from build123d import *

# Parameters (mm, degrees)
SKETCH_1_R          = 24
SKETCH_1_R_2        = 2
SKETCH_1_R_3        = 2.5
SKETCH_1_R_4        = 1.1
SKETCH_1_R_5        = 6
EXTRUDE_1_DEPTH     = 6
SKETCH_2_R          = 1
CUT_EXTRUDE_1_DEPTH = 84.432607534
FILLET_1_R          = 1


with BuildPart() as part:
    # 草图1 → 凸台-拉伸1 (new body)
    with BuildSketch(Plane.XY):
        with BuildLine():
            Line((-31, 0), (-31, 44.038518603))
            ThreePointArc((-31, 44.038518603), (-32.603168898, 47.707515532), (-36.384615385, 49.023703756))
            ThreePointArc((-36.384615385, 49.023703756), (-44.994071865, 56.692079518), (-37, 65))
            Line((-37, 65), (-12.5, 65))
            Line((-12.5, 65), (-12.5, 70))
            Line((-12.5, 70), (12.5, 70))
            Line((12.5, 70), (12.5, 65))
            Line((12.5, 65), (31, 65))
            Line((31, 65), (31, 0))
            ThreePointArc((31, 0), (24.191352338, -19.385006373), (6.756227609, -30.254807692))
            ThreePointArc((6.756227609, -30.254807692), (5.147421514, -30.170867126), (3.813999457, -29.266826923))
            ThreePointArc((3.813999457, -29.266826923), (0, -27.5), (-3.813999457, -29.266826923))
            ThreePointArc((-3.813999457, -29.266826923), (-5.147421514, -30.170867126), (-6.756227609, -30.254807692))
            ThreePointArc((-6.756227609, -30.254807692), (-24.191352338, -19.385006373), (-31, 0))
        make_face()
        Circle(SKETCH_1_R, mode=Mode.SUBTRACT)
        with Locations((-19.445436483, 19.445436483)):
            Circle(SKETCH_1_R_2, mode=Mode.SUBTRACT)
        with Locations((0, 27.5)):
            Circle(SKETCH_1_R_2, mode=Mode.SUBTRACT)
        with Locations((19.445436483, 19.445436483)):
            Circle(SKETCH_1_R_2, mode=Mode.SUBTRACT)
        with Locations((27.5, 0)):
            Circle(SKETCH_1_R_2, mode=Mode.SUBTRACT)
        with Locations((19.445436483, -19.445436483)):
            Circle(SKETCH_1_R_2, mode=Mode.SUBTRACT)
        with Locations((-19.445436483, -19.445436483)):
            Circle(SKETCH_1_R_2, mode=Mode.SUBTRACT)
        with Locations((-27.5, 0)):
            Circle(SKETCH_1_R_2, mode=Mode.SUBTRACT)
        with Locations((-26, 60)):
            Circle(SKETCH_1_R_3, mode=Mode.SUBTRACT)
        with Locations((0, 60)):
            Circle(SKETCH_1_R_3, mode=Mode.SUBTRACT)
        with Locations((26, 60)):
            Circle(SKETCH_1_R_3, mode=Mode.SUBTRACT)
        with Locations((-22.6, 50)):
            Circle(SKETCH_1_R_4, mode=Mode.SUBTRACT)
        with Locations((-22.6, 32)):
            Circle(SKETCH_1_R_4, mode=Mode.SUBTRACT)
        with Locations((22.6, 32)):
            Circle(SKETCH_1_R_4, mode=Mode.SUBTRACT)
        with Locations((22.6, 50)):
            Circle(SKETCH_1_R_4, mode=Mode.SUBTRACT)
        with Locations((-37, 57)):
            Circle(SKETCH_1_R_5, mode=Mode.SUBTRACT)
    extrude(amount=EXTRUDE_1_DEPTH)

    # 草图2 → 切除-拉伸1 (cut, through all)
    with BuildSketch(Plane.XY.offset(6)):
        with Locations((-13.5, 65)):
            Circle(SKETCH_2_R)
        with Locations((13.5, 65)):
            Circle(SKETCH_2_R)
    extrude(amount=-CUT_EXTRUDE_1_DEPTH, mode=Mode.SUBTRACT)

    # 圆角1
    fillet_1_edges = [part.edges().sort_by_distance(p)[0] for p in [
        (-12.5, 70, 3),
        (12.5, 70, 3),
        (31, 65, 3),
    ]]
    fillet(fillet_1_edges, radius=FILLET_1_R)


solid = part.part
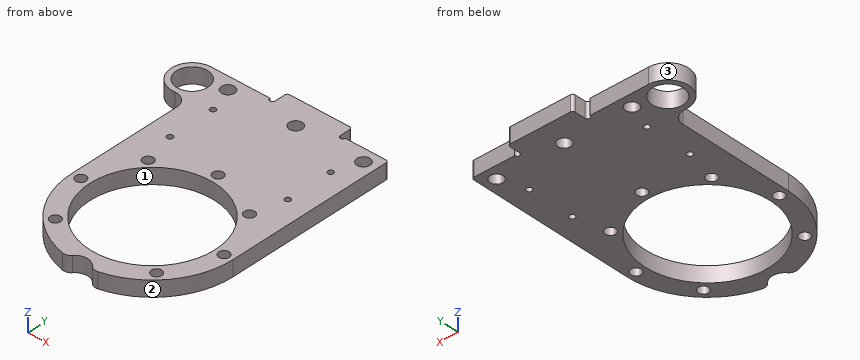
Input: part model. Units: mm. Frame: model coordinates. Face numbers are marked on the shaded views. Round coordinates to 2 decimals unless told otherwise and drop trailing zeros. Write each loop counter-clockwise with the first axis right and the second up, starting at its lowest first coordinate (ties: lowest second). Pieces come first, ordered by that corner, then holes.
1) Contact query for flat-ended pins moving along their axis: P1, Ø3, axis at x = -27.5, y = 0, coming from the -Z side; P2, Ø1.8, axis at x = -30, z = 2, coming from the +Y side; P3, Ø1, axis at x = -32, z = 1.5, coming from the -Y side; P4, Ø1, axis at y = 58.5, z = 2.5, coming from the -X side. Output: stop coordinate, or through.
2) Draft query along Y for the marked faces 1, 2 and 3. Return one class per face: pulls with the +Y half, pulls with the -Y half, needs draft (parallel to the pull), parting line crosses it, or undercut.
3) Cut plane C-C (x = -8.5). Return the cut outline in (y, z), then the cut area to 3 significant figures.
4) Cut plane D-D (y = 60). Return the cut outline in (x, z).
5) Cut plane B-B (x = 0). Return the cut outline in (y, z), then the cut area to 3 significant figures.
6) Cut plane A-A (y = 32). Return the cut outline in (x, z).
7) Ray query, L1, parallel to X at y = 21, z = 1.7; L2, parallel to Y at x = -18.5, z = 5.5; L3, parallel to X at y = 1, z = 5.6. Return the intervals inside material, ascending.
Geometry says:
1. P1: passes through
1. P2: stops at y = 65
1. P3: stops at y = 46.22
1. P4: stops at x = -44.94
2. face 1: undercut
2. face 2: pulls with the -Y half
2. face 3: parting line crosses it
3. outline: (-29.81, 0) - (-22.44, 0) - (-22.44, 6) - (-29.81, 6) - close; (22.44, 0) - (70, 0) - (70, 6) - (22.44, 6) - close
3. area: 330 mm2
4. outline: (-44.42, 0) - (-42.2, 0) - (-42.2, 6) - (-44.42, 6) - close; (-31.8, 0) - (-28.5, 0) - (-28.5, 6) - (-31.8, 6) - close; (-23.5, 0) - (-2.5, 0) - (-2.5, 6) - (-23.5, 6) - close; (2.5, 0) - (23.5, 0) - (23.5, 6) - (2.5, 6) - close; (28.5, 0) - (31, 0) - (31, 6) - (28.5, 6) - close
5. outline: (-27.5, 0) - (-24, 0) - (-24, 6) - (-27.5, 6) - close; (24, 0) - (25.5, 0) - (25.5, 6) - (24, 6) - close; (29.5, 0) - (57.5, 0) - (57.5, 6) - (29.5, 6) - close; (62.5, 0) - (70, 0) - (70, 6) - (62.5, 6) - close
5. area: 243 mm2
6. outline: (-31, 0) - (-23.7, 0) - (-23.7, 6) - (-31, 6) - close; (-21.5, 0) - (21.5, 0) - (21.5, 6) - (-21.5, 6) - close; (23.7, 0) - (31, 0) - (31, 6) - (23.7, 6) - close
7. L1: x = -31 to -20.7, -18.19 to -11.62, 11.62 to 18.19, 20.7 to 31
7. L2: y = -24.87 to -21.21, -17.68 to -15.29, 15.29 to 17.68, 21.21 to 65
7. L3: x = -31 to -29.23, -25.77 to -23.98, 23.98 to 25.77, 29.23 to 31
